```python
from build123d import *

# Parameters (mm, degrees)
SKETCH_2_W      = 200
SKETCH_2_H      = 120
EXTRUDE_1_DEPTH = 10
SKETCH_3_W      = 210
SKETCH_3_H      = 126
EXTRUDE_2_DEPTH = 3
SKETCH_8_W      = 120
SKETCH_8_H      = 80
EXTRUDE_4_DEPTH = 20
SKETCH_9_R      = 5
EXTRUDE_5_DEPTH = 2
SKETCH_10_R     = 2.5
EXTRUDE_6_DEPTH = 3


with BuildPart() as part:
    # 草图2 → 凸台-拉伸1 (new body)
    with BuildSketch(Plane.XY):
        Rectangle(SKETCH_2_W, SKETCH_2_H)
    extrude(amount=-EXTRUDE_1_DEPTH)

    # 草图3 → 凸台-拉伸2 (add)
    with BuildSketch(Plane(origin=(0, 0, -10), x_dir=(-1, 0, 0), z_dir=(0, 0, -1))):
        Rectangle(SKETCH_3_W, SKETCH_3_H)
    extrude(amount=EXTRUDE_2_DEPTH)

    # 草图5 → 放样2 section 0
    with BuildSketch(Plane(origin=(0, 0, -13), x_dir=(-1, 0, 0), z_dir=(0, 0, -1))):
        with BuildLine():
            Line((-100, 60), (100, 60))
            Line((100, 60), (100, -60))
            Line((100, -60), (-100, -60))
            Line((-100, -60), (-100, 60))
        make_face()
    # 草图4 → 放样2 section 1
    with BuildSketch(Plane(origin=(0, 0, -73), x_dir=(-1, 0, 0), z_dir=(0, 0, -1))):
        with BuildLine():
            Line((-60, 40), (60, 40))
            Line((60, 40), (60, -40))
            Line((60, -40), (-60, -40))
            Line((-60, -40), (-60, 40))
        make_face()
    loft()

    # 草图8 → 凸台-拉伸4 (add)
    with BuildSketch(Plane(origin=(0, 0, -73), x_dir=(-1, 0, 0), z_dir=(0, 0, -1))):
        Rectangle(SKETCH_8_W, SKETCH_8_H)
    extrude(amount=EXTRUDE_4_DEPTH)

    # 草图9 → 凸台-拉伸5 (add)
    with BuildSketch(Plane(origin=(60, 0, 0), x_dir=(0, 0, -1), z_dir=(1, 0, 0))):
        with Locations(Location((82.568018159, 0, 0), (0, 0, 180))):
            Circle(SKETCH_9_R)
    extrude_5 = extrude(amount=EXTRUDE_5_DEPTH)

    # 草图10 → 凸台-拉伸6 (add)
    with BuildSketch(Plane(origin=(62, 0, 0), x_dir=(0, 0, -1), z_dir=(1, 0, 0))):
        with Locations((82.568018159, 0)):
            Circle(SKETCH_10_R)
    extrude_6 = extrude(amount=EXTRUDE_6_DEPTH)

    # 镜向1: 凸台-拉伸5, 凸台-拉伸6 across plane
    add(extrude_5.mirror(Plane(origin=(0, 0, 0), x_dir=(0, 0, 1), z_dir=(1, 0, 0))))
    add(extrude_6.mirror(Plane(origin=(0, 0, 0), x_dir=(0, 0, 1), z_dir=(1, 0, 0))))


solid = part.part
```
Design review of the part built by this model. Coordinates are the model's own, in mm. A direction names the side the tool comes from. Coordinates: 2 decimals unless noted, no trailing zeros. Order: outer loops, then holes, each group sorted by start corner. A loop starts at its lowest first (then second) coordinate and runs counter-clockwise, first axis right, second up. Notation, with made-up numbers: (7.5, 57.5) -> (13.5, 57.5) arc R25 cw to (13.5, 88.5) -> close; hole circle Ø7 at (70.5, 18.25). An arc over 180 degrees is marked (long way). One line per item, written item: value. Start each with the question number.
Q1. Mouldability with a two-part tool opening along Z and no side actions: class faces 5 (the cylindrical face through (-63.48, 0.11, -80.07)), 6 (the flat face through (-1, 60, -5)), 7 (the flat face through (-1, 1, 0)) as pulls with the +Z half, pulls with the -Z half, needs draft (parallel to the pull), parting line crosses it, or undercut.
Q2. Insertion check: pin 1 Ø5 at (y, z) = (32.5, -55) entering from +X; pin 2 Ø8 at (y, z) = (47.5, -52) entering from -X; pin 3 Ø8 at (x, z) = (40.5, -5) entering from -Y. Each pin has a flat end and moves straight along its axis. Give the tip position at first contact, or say it passes through.
Q3. Tool access review of faces 1 (the flat face through (8.3, -60.4, -13)), 2 (the flat face through (65, 0, -83)), 3 (the cylindrical face through (-60.99, 1.92, -77.95)), 4 (the cylindrical face through (63.48, 0.11, -80.07)): name each direction out of +Z, -Z, +X, -X, +Y, -Y from which nothing blocks a thin tool from reaching the whole face with its end or side.
Q4. For probe 1 along X at (y, z) = (-0.5, -82.5); probe 2 along Y at (x, z) = (-13.5, -73); probe 3 along Y at (x, z) = (-55.5, -62.5), list the stretches that pass through material, from the lowest coordinate up.
Q5. Take a section at A-A, the plane z = -7. State the section outline as (x, y) points.
Values follow:
1. face 5: undercut
1. face 6: needs draft
1. face 7: pulls with the +Z half
2. pin 1: stops at x = 73.67
2. pin 2: stops at x = -76.67
2. pin 3: stops at y = -60
3. face 1: -Z
3. face 2: -Z, +X, +Y, -Y
3. face 3: -X
3. face 4: +X
4. probe 1: x = -65 to 65
4. probe 2: y = -40 to 40
4. probe 3: y = -43.5 to 43.5
5. outline: (-100, -60) -> (100, -60) -> (100, 60) -> (-100, 60) -> close
